Read the model definition and answer for the solid it produces. Units are mm, in the model's axes. A direction names the side the tool comes from. Give positions to 0.01 mm unless a question says otherwise; leave off trailing zeros. Write each loop counter-clockwise with the first axis right and the second up, starting at its lowest first coordinate (ties: lowest second). Pieces come first, ordered by that corner, then holes. Notation, with made-up numbers: M 64.5,5.25 L 100.5,5.25 A16 cw 100.5,20.25 Z; hole C 22.5,1 d2. An arc over 180 degrees is marked long. Use a Markdown table: item, result. Add a question column.
Item 1: For faces 1 (the flat face through (-6, -35, 82)), 2 (the flat face through (0, 37, 55)), 3 (the flat face through (0, -37, 55)), 4 (the flat face through (-4, 17, 99.5)), determine the directions among +Z, -Z, +X, -X, +Y, -Y from which every point of the face is accessible in a straight line to the end or side of a thin tool.
Item 2: A cutting plane is placed at B-B on z = 66. Determine the outline of the cut face in (x, y), then the cut area to 3 significant figures.
Item 3: The mould has two halves that part along Y. Classify faces 5 (the cylindrical face through (-5.9, 0.2, -12.5)), 6 (the cylindrical face through (-5.92, 56.92, 75.58)), 7 (the cylindrical face through (-5.916, 0.33, 7.493)), 8 (the flat face through (15.77, -16.92, 53.86)): pulls with the +Y half, pulls with the -Y half, needs draft (parallel to the pull), parting line crosses it, or undercut.
Item 4: A cutting plane is placed at C-C on x = 22.5. Determine the outline of the cut face in (y, z), then the cut area to 3 significant figures.
Item 5: Given P1, Ø19.5, axis at y = 46, z = 69.5, coming from the +X side; P2, Ø5, axis at x = -6, z = 99, coming from the -Y side; P3, Ø10, axis at y = -17, z = 60, coming from the +X side, each flat-ended and moving along its own axis, determine where each tip first touches the part or whether it passes through.
Item 6: A cutting plane is placed at D-D on x = -6. Determine the outline of the cut face in (y, z), then the cut area to 3 significant figures.
Item 7: Consider probe 1 along Y at (x, z) = (-3, 69); probe 2 along Y at (x, z) = (6.5, 43); probe 3 along X at (y, z) = (-14, 99). Determine where each line is inside the solid, lowest interval first. Write a range as [from, to].
Item 8: A cutting plane is placed at A-A on y = 0. Determine the outline of the cut face in (x, z).
from build123d import *

# Parameters (mm, degrees)
SKETCH1_R               = 7.5
BOSS_EXTRUDE1_DEPTH     = 12
SKETCH2_R               = 7.5
BOSS_EXTRUDE2_DEPTH     = 23
CUT_EXTRUDE1_REACH      = 132.347
SKETCH3_W               = 44
SKETCH3_H               = 22
CUT_EXTRUDE2_DEPTH      = 116.656819946
CUT_EXTRUDE2_DEPTH_BACK = 116.656819946
SKETCH4_W               = 28
SKETCH4_H               = 22
CUT_EXTRUDE3_DEPTH      = 116.656819946
CUT_EXTRUDE3_DEPTH_BACK = 116.656819946
SKETCH5_W               = 4
SKETCH5_H               = 22


with BuildPart() as part:
    # Sketch1 → Boss-Extrude1 (new body)
    with BuildSketch(Plane.YZ):
        with BuildLine():
            Line((-46, 82), (46, 82))
            ThreePointArc((46, 82), (57.011103253, 75.416553486), (56.423645014, 62.600896825))
            Line((56.423645014, 62.600896825), (10.423645014, -6.899103175))
            ThreePointArc((10.423645014, -6.899103175), (0, -12.5), (-10.423645014, -6.899103175))
            Line((-10.423645014, -6.899103175), (-56.423645014, 62.600896825))
            ThreePointArc((-56.423645014, 62.600896825), (-57.011103253, 75.416553486), (-46, 82))
        make_face()
        with Locations(Location((0, 0, 0), (0, 0, 270))):
            Circle(SKETCH1_R, mode=Mode.SUBTRACT)
        with Locations(Location((46, 69.5, 0), (0, 0, 270))):
            Circle(SKETCH1_R, mode=Mode.SUBTRACT)
        with Locations(Location((-46, 69.5, 0), (0, 0, 90))):
            Circle(SKETCH1_R, mode=Mode.SUBTRACT)
    extrude(amount=-BOSS_EXTRUDE1_DEPTH)

    # Sketch2 → Boss-Extrude2 (add, symmetric)
    with BuildSketch(Plane(origin=(0, 0, 0), x_dir=(-1, 0, 0), z_dir=(0, 1, 0))):
        with BuildLine():
            Line((12, 99.5), (-4, 99.5))
            ThreePointArc((-4, 99.5), (-20.50814275, 113.273497012), (-31.101317135, 94.564871904))
            Line((-31.101317135, 94.564871904), (0, 12))
            Line((0, 12), (0, 82))
            Line((0, 82), (12, 82))
            Line((12, 82), (12, 99.5))
        make_face()
        with Locations(Location((-18, 99.5, 0), (0, 0, 90))):
            Circle(SKETCH2_R, mode=Mode.SUBTRACT)
    extrude(amount=BOSS_EXTRUDE2_DEPTH, both=True)

    # Cut-Extrude1: up to this face of the body (flat: up to its plane)
    cut_extrude1_end = Plane(part.part.faces().sort_by_distance((-6, -34.5, 82))[0])
    # Sketch3 → Cut-Extrude1 (cut, up to the picked face)
    with BuildSketch(Plane.XY.offset(99.5), mode=Mode.PRIVATE) as cut_extrude1_sk1:
        with Locations((10, 0)):
            Rectangle(SKETCH3_W, SKETCH3_H)
    cut_extrude1_tool1 = split(extrude(cut_extrude1_sk1.sketch, amount=-CUT_EXTRUDE1_REACH, mode=Mode.PRIVATE), bisect_by=cut_extrude1_end, keep=Keep.BOTH, mode=Mode.PRIVATE)
    add(cut_extrude1_tool1.solids().sort_by(Axis((10, 0, 99.5), (0, 0, -1)))[0], mode=Mode.SUBTRACT)

    # Sketch4 → Cut-Extrude2 (cut, two sides: drawn at the far end of the back side and taken through both)
    with BuildSketch(Plane.XY.offset(82).offset(-CUT_EXTRUDE2_DEPTH_BACK)):
        with Locations((18, 0)):
            Rectangle(SKETCH4_W, SKETCH4_H)
    extrude(amount=CUT_EXTRUDE2_DEPTH + CUT_EXTRUDE2_DEPTH_BACK, mode=Mode.SUBTRACT)

    # Sketch5 → Cut-Extrude3 (cut, two sides: drawn at the far end of the back side and taken through both)
    with BuildSketch(Plane.XY.offset(82).offset(-CUT_EXTRUDE3_DEPTH_BACK)):
        with Locations((2, 0)):
            Rectangle(SKETCH5_W, SKETCH5_H)
    extrude(amount=CUT_EXTRUDE3_DEPTH + CUT_EXTRUDE3_DEPTH_BACK, mode=Mode.SUBTRACT)


solid = part.part
Filled in:
| question | item | result |
|---|---|---|
| 1 | face 1 | +Z, +X, -X, -Y |
| 1 | face 2 | +Z, -Z, +X, +Y |
| 1 | face 3 | +Z, -Z, +X, -Y |
| 1 | face 4 | +Z, -X, +Y, -Y |
| 2 | outline | M -12,-58 L 0,-58 L 0,-52.63 L -12,-52.63 Z; M -12,-39.37 L 0,-39.37 L 0,-23 L 20.34,-23 L 20.34,-11 L 0,-11 L 0,11 L 20.34,11 L 20.34,23 L 0,23 L 0,39.37 L -12,39.37 Z; M -12,52.63 L 0,52.63 L 0,58 L -12,58 Z |
| 2 | area | 1,560 mm² |
| 3 | face 5 | parting line crosses it |
| 3 | face 6 | pulls with the +Y half |
| 3 | face 7 | undercut |
| 3 | face 8 | needs draft |
| 4 | outline | M -23,71.73 L -11,71.73 L -11,93.5 L -23,93.5 Z; M -23,105.5 L -11,105.5 L -11,112.76 L -23,112.76 Z; M 11,71.73 L 23,71.73 L 23,93.5 L 11,93.5 Z; M 11,105.5 L 23,105.5 L 23,112.76 L 11,112.76 Z |
| 4 | area | 697 mm² |
| 5 | P1 | x = 0 |
| 5 | P2 | y = -23 |
| 5 | P3 | x = 19.96 |
| 6 | outline | M -56.42,62.6 L -10.42,-6.9 A12.5 ccw 10.42,-6.9 L 56.42,62.6 A12.5 ccw 46,82 L 23,82 L 23,99.5 L 11,99.5 L 11,82 L -11,82 L -11,99.5 L -23,99.5 L -23,82 L -46,82 A12.5 ccw Z; hole C -46,69.5 d15; hole C 0,0 d15; hole C 46,69.5 d15 |
| 6 | area | 6,810 mm² |
| 7 | probe 1 | [-58.49, -53.48], [-38.52, 38.52], [53.48, 58.49] |
| 7 | probe 2 | [-23, -11], [11, 23] |
| 7 | probe 3 | [-12, 10.52], [25.48, 31.99] |
| 8 | outline | M -12,-12.5 L 0,-12.5 L 0,-7.5 L -12,-7.5 Z; M -12,7.5 L 0,7.5 L 0,82 L -12,82 Z |
